Autodesk Inventor part; units mm, degrees
ref_plane "YZ Plane" through (0, 0, 0) normal (1, 0, 0) x (0, 1, 0)
ref_plane "XZ Plane" through (0, 0, 0) normal (0, 1, 0) x (-1, 0, 0)
ref_plane "XY Plane" through (0, 0, 0) normal (0, 0, 1) x (1, 0, 0)
sketch "Эскиз1" plane through (0, 0, 0) normal (0, 1, 0) x (-1, 0, 0)
  circle A0 centre (0, 0) radius 6
  circle A1 centre (0, 0) radius 4.4
  dimension "d6" = 12
  dimension "d7" = 8.8
extrude "Выдавливание1" add sketch "Эскиз1" along normal blind 5
sketch "Эскиз2" plane through (0, 5, 0) normal (0, 1, 0) x (1, 0, 0)
  circle A0 centre (0, 0) radius 4.4
  arc A1 (2.2, 3.8105) -> (0, 4.4) centre (0, 0) ccw
  line L0 (0, 0) -> (2.2, 3.8105) construction
  line L1 (0, 0) -> (0, 4.4) construction
  line L2 (2.2, 3.8105) -> (3.5243, 6.4533)
  line L3 (0, 4.4) -> (0, 6.8034)
  circle A2 centre (0, 0) radius 6
  point P0 (2.9177, 5.2428)
  point P1 (0, 6)
  dimension "d8" = 30
extrude "Выдавливание2" cut sketch "Эскиз2" against normal blind 5 contours A0 L3 A2 L2 picked at (0.3369, 5.4381)
fillet "Сопряжение2" radius 0.5 2 edges at (-1.1388, 0, 4.2501) (-1.1388, 5, 4.2501)
properties part number "fittingRingInstalled" material "Пластик ПАЭК"
Design review of the part built by this model. Coordinates are the model's own, in mm. A direction names the side the tool comes from. Round coordinates to 2 decimals unless told otherwise and drop trailing zeros. Write each loop counter-clockwise with the first axis right and the second up, starting at its lowest first coordinate (ties: lowest second). Pieces come first, ordered by that corner, then holes. Notation, with made-up numbers: (41.25, 55.5) - (65.25, 55.5) arc R22 cw to (65.25, 67.5) - close; hole circle Ø5 at (-13.75, -4). An arc over 180 degrees is marked (long way). Return JSON: item names as keys, results as strings. Group by question number.
Item 1: Machinability: for faces 4 (the face through (0, 3, -5)), 5 (the face through (-1, 0, 5)), which of the approach directions +Z, -Z, +X, -X, +Y, -Y give a long, thin tool a straight path to every point of the face, cutting with its end or side? Answer none if there is none.
Item 2: We need section A-A on z = 0. Write out the cut boundary in (x, y).
Item 3: For probe 1 along X at (y, z) = (2.95, 0); probe 2 along X at (y, z) = (0.45, 2.5); probe 3 along Z at (x, y) = (-1.5, 3.4), list the stretches that pass through material, from the lowest coordinate up. Write a range as [from, to].
Item 4: We need section B-B on y = 4.2. Write out the cut boundary in (x, z).
Item 5: The part is to be moulded in two halves that separate along X. For faces 1 (the face through (-1.271, 2.465, 5.864)), 2 (the face through (-0.97, 2.47, 4.29)), 3 (the face through (-1, 5, 5)), say which applies: pulls with the +X half, pulls with the -X half, needs draft (parallel to the pull), parting line crosses it, or undercut.
Item 6: Insertion check: P1, Ø1.5, axis at y = 3.5, z = 4.5, coming from the +X side; P2, Ø1.5, axis at y = 2, z = -3.5, coming from the -X side. Each pin has a flat end and moves straight along its axis. Give the tip position at first contact, or say it passes through.
Model answer:
{
 "1": {"face 4": "-Z, +Y, -Y", "face 5": "+Z, -Z, +X, -X, -Y"},
 "2": {"outline": "(-6, 0) - (-4.9, 0) arc R0.5 ccw to (-4.4, 0.5) - (-4.4, 4.5) arc R0.5 ccw to (-4.9, 5) - (-6, 5) - close; (4.4, 0.5) arc R0.5 ccw to (4.9, 0) - (6, 0) - (6, 5) - (4.9, 5) arc R0.5 ccw to (4.4, 4.5) - close"},
 "3": {"probe 1": "x = [-6, -4.4], [4.4, 6]", "probe 2": "x = [-5.45, -3.62], [3.62, 5.45]", "probe 3": "z = [-5.81, -4.14], [4.14, 5.81]"},
 "4": {"outline": "(0, -6) - (0, -4.4) arc R4.4 cw (long way) to (2.2, -3.81) - (2.92, -5.24) arc R6 ccw (long way) to start"},
 "5": {"face 1": "parting line crosses it", "face 2": "undercut", "face 3": "needs draft"},
 "6": {"P1": "stops at x = 4.68", "P2": "stops at x = -5.33"}
}
